```python
from build123d import *

# Parameters (mm, degrees)
SKETCH_1_R               = 7.5
EXTRUDE_1_DEPTH          = 150
SKETCH_2_R               = 10
EXTRUDE_2_DEPTH          = 29
CUT_EXTRUDE_1_DEPTH      = 180.55779014
CUT_EXTRUDE_1_DEPTH_BACK = 180.55779014
SKETCH_3_R               = 3.25


with BuildPart() as part:
    # 草图1 → 凸台-拉伸1 (new body)
    with BuildSketch(Plane(origin=(0, 0, 0), x_dir=(1, 0, 0), z_dir=(0, 1, 0))):
        with Locations(Location((0, 0, 0), (0, 0, 270))):
            Circle(SKETCH_1_R)
    extrude(amount=EXTRUDE_1_DEPTH)

    # 草图2 → 凸台-拉伸2 (add)
    with BuildSketch(Plane(origin=(0, 150, 0), x_dir=(1, 0, 0), z_dir=(0, 1, 0))):
        with Locations(Location((0, 0, 0), (0, 0, 90))):
            Circle(SKETCH_2_R)
    extrude(amount=EXTRUDE_2_DEPTH)

    # 草图3 → 切除-拉伸1 (cut, two sides: drawn at the far end of the back side and taken through both)
    with BuildSketch(Plane.XY.offset(-CUT_EXTRUDE_1_DEPTH_BACK)):
        with Locations(Location((0, 170, 0), (0, 0, 89.999999989))):
            Circle(SKETCH_3_R)
    extrude(amount=CUT_EXTRUDE_1_DEPTH + CUT_EXTRUDE_1_DEPTH_BACK, mode=Mode.SUBTRACT)


solid = part.part
```
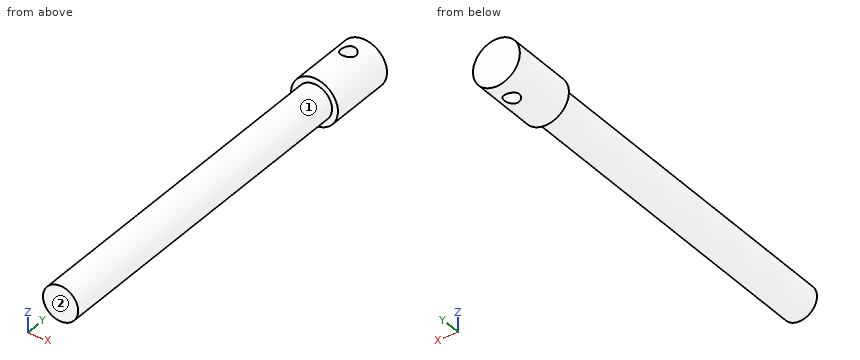
CAD build for the part. Positions are in the model's coordinates, mm. Face numbers are marked on the shaded views. A direction names the side the tool comes from. Round coordinates to 2 decimals unless told otherwise and drop trailing zeros. Write each loop counter-clockwise with the first axis right and the second up, starting at its lowest first coordinate (ties: lowest second). Pieces come first, ordered by that corner, then holes.
Item 1: Tool access for the marked faces 1 and 2: list every direction of +Z, -Z, +X, -X, +Y, -Y with a clear straight run to the whole face (end or side of a thin tool).
Filled in:
face 1: -Y
face 2: +Z, -Z, +X, -X, -Y
Item 2: Band-saw the part on B-B on z = 0. Write the cut outline in (x, y), then the cut area to 3 significant figures.
Filled in:
outline: (-10, 150) - (-7.5, 150) - (-7.5, 0) - (7.5, 0) - (7.5, 150) - (10, 150) - (10, 179) - (-10, 179) - close; hole circle Ø6.5 at (0, 170)
area: 2,800 mm2
Item 3: Band-saw the part on C-C on y = 170. Write the cut outline in (x, z).
Filled in:
outline: (-3.25, -9.46) - (-3.25, 9.46) arc R10 ccw to start; (3.25, -9.46) arc R10 ccw to (3.25, 9.46) - close
Item 4: Drop flat-ended pins along their axis: pin 1 Ø6 at (y, z) = (68, 1.5) entering from -X; pin 2 Ø8 at (x, y) = (6.5, 147.5) entering from -Z; pin 3 Ø10 at (y, z) = (114, -5.5) entering from +X. Give the stop position or say it passes through.
Filled in:
pin 1: stops at x = -7.5
pin 2: stops at z = -9.41
pin 3: stops at x = 7.48
Item 5: Drill centre lines: L1, parallel to X at y = 170, z = -0.25; L2, parallel to Y at x = 2.25, z = -3.25; L3, parallel to Y at x = -7, z = -6.5. Where is each one in solid material? Low to high.
Filled in:
L1: x = -10 to -3.25, 3.25 to 10
L2: y = 0 to 167.65, 172.35 to 179
L3: y = 150 to 179
Item 6: Band-saw the part on A-A on x = 0. Write the cut outline in (y, z).
Filled in:
outline: (0, -7.5) - (150, -7.5) - (150, -10) - (166.75, -10) - (166.75, 10) - (150, 10) - (150, 7.5) - (0, 7.5) - close; (173.25, -10) - (179, -10) - (179, 10) - (173.25, 10) - close
Item 7: Band-saw the part on D-D on y = 118. Write the cut outline in (x, z).
Filled in:
outline: circle Ø15 at (0, 0)
